The model under review builds one solid part; all positions refer to its coordinate system, in mm. Face numbers are marked on the shaded views. Round coordinates to 2 decimals unless told otherwise and drop trailing zeros. Order: outer loops, then holes, each group sorted by start corner. A loop starts at its lowest first (then second) coordinate and runs counter-clockwise, first axis right, second up. Notation, with made-up numbers: M 50,13 L 92,13 A31 cw 92,41 Z; hole C 2.5,26 d9. An arc over 180 degrees is marked long. Answer as a JSON object with one key per item and string values. Group by question number.
1. Add section A-A on y = 8.5. State the section outline as (x, z) points, and give its area (3 significant figures).
2. Add section C-C on x = 1. State the section outline as (y, z) points.
3. Add section D-D on x = 22.5. State the section outline as (y, z) points.
4. Clearance check with flat-ended pins moving along their axes: P1, Ø1.5, axis at x = -24, y = 5.5, coming from the +Z side; P2, Ø6, axis at y = 5.5, z = -6.5, coming from the -X side; P3, Ø25, axis at x = 10, z = 12.5, coming from the +Y side. State where each tip first meets the part, or that it passes through.
5. To check wall thickness, follow probe 1 along X at (y, z) = (5.75, -20); probe 2 along Y at (x, z) = (21.5, 3.5); probe 3 along Z at (x, y) = (-23, 0.25). State the ranges of each line that lie inside material, in increasing order. Write a range as [from, to].
6. Mouldability with a two-part tool opening along X and no side actions: class the marked faces 1, 2, 3 and 4 as released by +X, released by -X, zero draft, split by the parting line, or undercut.
7. Add section B-B on z = -20. State the section outline as (x, y) points.
```python
from build123d import *

# Parameters (mm, degrees)
SKETCH1_W           = 60
SKETCH1_H           = 80
BOSS_EXTRUDE2_DEPTH = 5
SKETCH1_7_R         = 5.2
BOSS_EXTRUDE4_DEPTH = 12
CHAMFER1_SIZE       = 5


with BuildPart() as part:
    # Sketch1 → Boss-Extrude2 (new body)
    with BuildSketch(Plane(origin=(0, 0, 0), x_dir=(1, 0, 0), z_dir=(0, 1, 0))):
        Rectangle(SKETCH1_W, SKETCH1_H)
    extrude(amount=-BOSS_EXTRUDE2_DEPTH)

    # Sketch1<7> → Boss-Extrude4 (add)
    with BuildSketch(Plane(origin=(0, 0, 0), x_dir=(1, 0, 0), z_dir=(0, 1, 0))):
        with BuildLine():
            Line((-15.656226575, 14.951726095), (-13.904483467, 17.118101406))
            ThreePointArc((-13.904483467, 17.118101406), (8.928488267, 31.041833963), (0.092207471, 5.800299377))
            Line((0.092207471, 5.800299377), (-1.659535637, 3.633924066))
            ThreePointArc((-1.659535637, 3.633924066), (9.580000014, 6.627412377), (16.03, 16.306546332))
            ThreePointArc((16.03, 16.306546332), (29.95, 20), (16.03, 23.693453668))
            ThreePointArc((16.03, 23.693453668), (0, 36.45), (-16.03, 23.693453668))
            ThreePointArc((-16.03, 23.693453668), (-29.95, 20), (-16.03, 16.306546332))
            ThreePointArc((-16.03, 16.306546332), (-15.857588818, 15.625142644), (-15.656226575, 14.951726095))
        make_face()
        with Locations(Location((-22.5, 20, 0), (0, 0, 270))):
            Circle(SKETCH1_7_R, mode=Mode.SUBTRACT)
        with Locations(Location((22.5, 20, 0), (0, 0, 270))):
            Circle(SKETCH1_7_R, mode=Mode.SUBTRACT)
    extrude(amount=BOSS_EXTRUDE4_DEPTH)

    # Chamfer1
    # the kernel refuses this chamfer: 5 mm, written as the material it takes off along each edge
    with BuildSketch(Plane(origin=(42.85841494, 0, -40), x_dir=(0, 0.027495876610586372, 0.9996219169112968), z_dir=(-1, 0, 0))) as chamfer1_piece_1_section:
        Polygon((CHAMFER1_SIZE * 0.999621916911, -CHAMFER1_SIZE * 0.0274958766106), (-CHAMFER1_SIZE * 0.0274958766106, -CHAMFER1_SIZE * 0.999621916911), (0, 0), align=None)
    chamfer1_piece_1 = extrude(amount=85.71682988, mode=Mode.PRIVATE)
    chamfer1_piece_1 = chamfer1_piece_1 - Plane(origin=(0, -1.679599763, -20), x_dir=(0.9744680851063817, 0, -0.22452605886422566), z_dir=(0, -1, 0)) * Cylinder(16.45, 192, mode=Mode.PRIVATE)
    add(chamfer1_piece_1, mode=Mode.SUBTRACT)
    with BuildSketch(Plane(origin=(30, 0, 52.85841494), x_dir=(0.027495876610586317, -0.9996219169112968, 0), z_dir=(0, 0, -1))) as chamfer1_piece_2_section:
        Polygon((CHAMFER1_SIZE * 0.999621916911, CHAMFER1_SIZE * 0.0274958766106), (-CHAMFER1_SIZE * 0.0274958766106, CHAMFER1_SIZE * 0.999621916911), (0, 0), align=None)
    chamfer1_piece_2 = extrude(amount=105.71682988, mode=Mode.PRIVATE)
    chamfer1_piece_2 = chamfer1_piece_2 - Plane(origin=(22.5, -1.692858266, -20), x_dir=(-0.8684563758389187, 0, 0.49576559306261964), z_dir=(0, -1, 0)) * Cylinder(7.45, 232, mode=Mode.PRIVATE)
    add(chamfer1_piece_2, mode=Mode.SUBTRACT)
    with BuildSketch(Plane(origin=(-42.85841494, 0, 40), x_dir=(0, -0.9996219169112968, 0.027495876610586317), z_dir=(1, 0, 0))) as chamfer1_piece_3:
        Polygon((CHAMFER1_SIZE * 0.999621916911, CHAMFER1_SIZE * 0.0274958766106), (-CHAMFER1_SIZE * 0.0274958766106, CHAMFER1_SIZE * 0.999621916911), (0, 0), align=None)
    extrude(amount=85.71682988, mode=Mode.SUBTRACT)
    with BuildSketch(Plane(origin=(-30, 0, -52.85841494), x_dir=(-0.027495876610586317, -0.9996219169112968, 0), z_dir=(0, 0, 1))) as chamfer1_piece_4_section:
        Polygon((CHAMFER1_SIZE * 0.999621916911, CHAMFER1_SIZE * 0.0274958766106), (-CHAMFER1_SIZE * 0.0274958766106, CHAMFER1_SIZE * 0.999621916911), (0, 0), align=None)
    chamfer1_piece_4 = extrude(amount=105.71682988, mode=Mode.PRIVATE)
    chamfer1_piece_4 = chamfer1_piece_4 - Plane(origin=(-22.5, -1.692858266, -20), x_dir=(0.8684563758389191, 0, -0.4957655930626189), z_dir=(0, -1, 0)) * Cylinder(7.45, 232, mode=Mode.PRIVATE)
    add(chamfer1_piece_4, mode=Mode.SUBTRACT)


solid = part.part
```
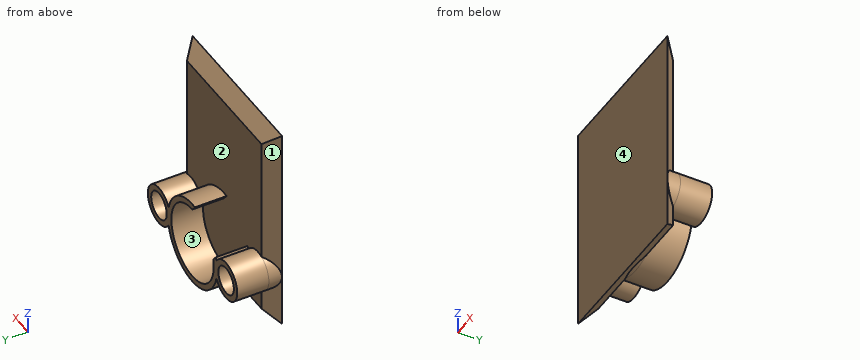
Recorded:
{
 "1": {"outline": "M -16.03,-23.69 A16.45 ccw 16.03,-23.69 A7.45 ccw long 16.03,-16.31 A16.45 ccw -1.66,-3.63 L 0.09,-5.8 A14.2 cw long -13.9,-17.12 L -15.66,-14.95 A16.45 ccw -16.03,-16.31 A7.45 ccw long Z; hole C -22.5,-20 d10.4; hole C 22.5,-20 d10.4", "area": "338 mm²"},
 "2": {"outline": "M -5,-40 L -1.42,-36.42 L 12,-36.42 L 12,-34.16 L 0,-34.16 L 0,-5.84 L 12,-5.84 L 12,-3.58 L 0,-3.58 L 0,35 L -5,40 Z"},
 "3": {"outline": "M -5,-40 L 0,-35 L 0,-27.45 L 12,-27.45 L 12,-25.2 L 0,-25.2 L 0,-14.8 L 12,-14.8 L 12,-12.55 L 0,-12.55 L 0,35 L -5,40 Z"},
 "4": {"P1": "stops at z = -12.59", "P2": "stops at x = -1.66", "P3": "stops at y = 0"},
 "5": {"probe 1": "x = [-29.95, -27.7], [-17.3, -14.2], [14.2, 17.3], [27.7, 29.95]", "probe 2": "y = [-5, 0]", "probe 3": "z = [-27.43, -25.18], [-14.82, -12.57]"},
 "6": {"face 1": "released by -X", "face 2": "undercut", "face 3": "undercut", "face 4": "zero draft"},
 "7": {"outline": "M -30,-5 L 30,-5 L 29.95,-4.95 L 29.95,12 L 27.7,12 L 27.7,0 L 17.3,0 L 17.3,12 L 14.2,12 L 14.2,0 L -14.2,0 L -14.2,12 L -17.3,12 L -17.3,0 L -27.7,0 L -27.7,12 L -29.95,12 L -29.95,-4.95 Z"}
}
